```python
from build123d import *

# Parameters (mm, degrees)
EXTRUDE_1_DEPTH     = 3
SKETCH_2_W          = 4
SKETCH_2_H          = 25
EXTRUDE_2_DEPTH     = 3
SKETCH_6_R          = 1.6
CUT_EXTRUDE_4_DEPTH = 4
CUT_EXTRUDE_5_DEPTH = 10
CUT_EXTRUDE_7_DEPTH = 10
FILLET_1_R          = 5
SKETCH_11_R         = 1.5
CUT_EXTRUDE_8_DEPTH = 90.117899437


with BuildPart() as part:
    # 草图1 → 凸台-拉伸1 (new body)
    with BuildSketch(Plane(origin=(0, 0, 0), x_dir=(0, 0, -1), z_dir=(1, 0, 0))):
        Polygon((-46, -23), (-68, 40), (-74, 40), (-74, -20.726707409), (-61, -40), (-61, -43), (-31, -43), (-31, -40), (19, -40), (19, -43), (49, -43), (49, -40), (74, -2.935975787), (74, 40), (68, 40), (34, -23), align=None)
    extrude(amount=EXTRUDE_1_DEPTH)

    # 草图2 → 凸台-拉伸2 (add)
    with BuildSketch(Plane(origin=(3, 0, 0), x_dir=(0, 0, -1), z_dir=(1, 0, 0))):
        with Locations((-76, 17.5)):
            Rectangle(SKETCH_2_W, SKETCH_2_H)
        with Locations((76, 17.5)):
            Rectangle(SKETCH_2_W, SKETCH_2_H)
    extrude(amount=-EXTRUDE_2_DEPTH)

    # 草图6 → 切除-拉伸4 (cut)
    with BuildSketch(Plane.ZY):
        with Locations((-71, 5)):
            Circle(SKETCH_6_R)
        with Locations((71, 25)):
            Circle(SKETCH_6_R)
        with Locations((71, 5)):
            Circle(SKETCH_6_R)
        with Locations((-71, 25)):
            Circle(SKETCH_6_R)
    extrude(amount=-CUT_EXTRUDE_4_DEPTH, mode=Mode.SUBTRACT)

    # 草图7 → 切除-拉伸5 (cut)
    with BuildSketch(Plane(origin=(3, 0, 0), x_dir=(0, 0, -1), z_dir=(1, 0, 0))):
        with BuildLine():
            Line((-66, 13.209781141), (-66, -4.624153975))
            ThreePointArc((-66, -4.624153975), (-65.936068557, -4.975971621), (-65.752448687, -5.282804848))
            Line((-65.752448687, -5.282804848), (-55.391275304, -17.119502604))
            ThreePointArc((-55.391275304, -17.119502604), (-54.135455337, -17.324921956), (-53.694734868, -16.131168898))
            Line((-53.694734868, -16.131168898), (-64.055908251, 13.539463974))
            ThreePointArc((-64.055908251, 13.539463974), (-65.167194873, 14.195705009), (-66, 13.209781141))
        make_face()
        with BuildLine():
            Line((66, -4.449930151), (66, 21.807804944))
            ThreePointArc((66, 21.807804944), (65.244926343, 22.777346633), (64.119977827, 22.282737545))
            Line((64.119977827, 22.282737545), (42.579599238, -17.630316899))
            ThreePointArc((42.579599238, -17.630316899), (42.777733508, -18.836706189), (43.995039468, -18.94983668))
            Line((43.995039468, -18.94983668), (65.535418057, -5.29451733))
            ThreePointArc((65.535418057, -5.29451733), (65.876190064, -4.931895887), (66, -4.449930151))
        make_face()
        Polygon((-74, 0), (-61, -40), (-74, -20.726707409), align=None)
        with BuildLine():
            Line((-62.213350607, -13.880667443), (-52.307335811, -25.197387929))
            ThreePointArc((-52.307335811, -25.197387929), (-52.061835208, -25.920048281), (-52.39764858, -26.605422566))
            Line((-52.39764858, -26.605422566), (-57.236264859, -30.880697516))
            ThreePointArc((-57.236264859, -30.880697516), (-58.161708676, -31.096025601), (-58.849434846, -30.440399824))
            Line((-58.849434846, -30.440399824), (-63.916833363, -14.848404388))
            ThreePointArc((-63.916833363, -14.848404388), (-63.459750443, -13.669828659), (-62.213350607, -13.880667443))
        make_face()
        with BuildLine():
            Line((-55.387669494, -33.250616236), (-49.831358953, -28.341205383))
            ThreePointArc((-49.831358953, -28.341205383), (-49.414538234, -28.121145774), (-48.943216882, -28.116463272))
            Line((-48.943216882, -28.116463272), (-27.782801194, -33.025874126))
            ThreePointArc((-27.782801194, -33.025874126), (-27.015296935, -34.11374121), (-28.008807346, -35))
            Line((-28.008807346, -35), (-54.725533576, -35))
            ThreePointArc((-54.725533576, -35), (-55.660783212, -34.353988867), (-55.387669494, -33.250616236))
        make_face()
        with BuildLine():
            Line((-23.126212383, -29), (11.126212383, -29))
            ThreePointArc((11.126212383, -29), (12.119722794, -29.88625879), (11.352218536, -30.974125874))
            Line((11.352218536, -30.974125874), (-5.773993847, -34.947564496))
            ThreePointArc((-5.773993847, -34.947564496), (-6, -34.973438622), (-6.226006153, -34.947564496))
            Line((-6.226006153, -34.947564496), (-23.352218536, -30.974125874))
            ThreePointArc((-23.352218536, -30.974125874), (-24.119722794, -29.88625879), (-23.126212383, -29))
        make_face()
        with BuildLine():
            Line((15.782801194, -33.025874126), (36.943216882, -28.116463272))
            ThreePointArc((36.943216882, -28.116463272), (37.414538234, -28.121145774), (37.831358953, -28.341205383))
            Line((37.831358953, -28.341205383), (43.387669494, -33.250616236))
            ThreePointArc((43.387669494, -33.250616236), (43.660783212, -34.353988867), (42.725533576, -35))
            Line((42.725533576, -35), (16.008807346, -35))
            ThreePointArc((16.008807346, -35), (15.015296935, -34.11374121), (15.782801194, -33.025874126))
        make_face()
        with BuildLine():
            Line((40.32049134, -24.831312908), (58.783941471, -13.126583263))
            ThreePointArc((58.783941471, -13.126583263), (60.036438838, -13.274178861), (60.148397101, -14.530363346))
            Line((60.148397101, -14.530363346), (48.30691143, -32.086087811))
            ThreePointArc((48.30691143, -32.086087811), (47.604393348, -32.518859029), (46.815737939, -32.276278671))
            Line((46.815737939, -32.276278671), (40.193773479, -26.425283852))
            ThreePointArc((40.193773479, -26.425283852), (39.859054482, -25.596651891), (40.32049134, -24.831312908))
        make_face()
    extrude(amount=-CUT_EXTRUDE_5_DEPTH, mode=Mode.SUBTRACT)

    # 草图10 → 切除-拉伸7 (cut)
    with BuildSketch(Plane.ZY):
        with BuildLine():
            Line((61.096725602, -39.702382762), (61, -40.312940669))
            ThreePointArc((61, -40.312940669), (61, -40), (61.096725602, -39.702382762))
        make_face()
        with BuildLine():
            Line((-74, 30), (-74, 32))
            ThreePointArc((-74, 32), (-73, 31), (-74, 30))
        make_face()
        with BuildLine():
            Line((74, 30), (74, 32))
            ThreePointArc((74, 32), (73, 31), (74, 30))
        make_face()
        with BuildLine():
            Line((-74, 3.585786438), (-75.414213562, 5))
            ThreePointArc((-75.414213562, 5), (-74, 5), (-74, 3.585786438))
        make_face()
        with BuildLine():
            Line((74, 3.585786438), (75.414213562, 5))
            ThreePointArc((75.414213562, 5), (74, 5), (74, 3.585786438))
        make_face()
        with BuildLine():
            Line((-17, -40), (-19, -40))
            ThreePointArc((-19, -40), (-18, -39), (-17, -40))
        make_face()
        with BuildLine():
            Line((29, -40), (31, -40))
            ThreePointArc((31, -40), (30, -39), (29, -40))
        make_face()
        with BuildLine():
            Line((-49.326984365, -39.515225743), (-49, -40.584743409))
            ThreePointArc((-49, -40.584743409), (-49, -40), (-49.326984365, -39.515225743))
        make_face()
    extrude(amount=-CUT_EXTRUDE_7_DEPTH, mode=Mode.SUBTRACT)

    # 圆角1
    fillet_1_edges = [part.edges().sort_by_distance(p)[0] for p in [
        (1.5, -23, 46),
        (1.5, -23, -34),
    ]]
    fillet(fillet_1_edges, radius=FILLET_1_R)

    # 草图11 → 切除-拉伸8 (cut, through all)
    with BuildSketch(Plane(origin=(3, 0, 0), x_dir=(0, 0, -1), z_dir=(1, 0, 0))):
        with Locations((-1, -26)):
            Circle(SKETCH_11_R)
        with Locations((-21, -26)):
            Circle(SKETCH_11_R)
    extrude(amount=-CUT_EXTRUDE_8_DEPTH, mode=Mode.SUBTRACT)


solid = part.part
```
Work out the finished part from the listing and answer in its coordinate system (mm). A direction names the side the tool comes from. Coordinates: 2 decimals unless noted, no trailing zeros. Loops run counter-clockwise (first coordinate to the right, second up) from the corner with the lowest first, then second, coordinate; pieces in that order, holes last. Notation, with made-up numbers: (29.5, -22.5) - (37.5, -22.5) arc R14 ccw to (37.5, 1.5) - close; hole circle Ø5 at (84, 74). An arc over 180 degrees is marked (long way). Use a Markdown table: item, result.
Item 1: For faces 1 (the cylindrical face through (1.52, -22.05, 45.38)), 2 (the flat face through (2, 30, -76)), 3 (the flat face through (1, 0, -74)), 4 (the flat face through (1.521, -30.606, -26.215)), 5 (the flat face through (2, 30, 76)), determine the directions among +Z, -Z, +X, -X, +Y, -Y from which every point of the face is accessible in a straight line to the end or side of a thin tool.
Evaluation:
| item | result |
|---|---|
| face 1 | +X, -X, +Y |
| face 2 | -Z, +X, -X, +Y |
| face 3 | -Z, +X, -X, -Y |
| face 4 | +X, -X |
| face 5 | +Z, +X, -X, +Y |
Item 2: Consider probe 1 along Z at (x, y) = (1.75, 16); probe 2 along Y at (x, z) = (1.85, -71); probe 3 along Y at (x, z) = (1.15, -37). Determine where each line is inside the solid, lowest interval first. Write a range as from..to.
Evaluation:
| item | result |
|---|---|
| probe 1 | z = -78..-66, -60.73..-55.05, 59.62..78 |
| probe 2 | y = -7.38..3.4, 6.6..23.4, 26.6..40 |
| probe 3 | y = -43..-35, -28.11..-17.44 |
Item 3: Find section C-C, the plane x = 0.7. State how many separate pieces and enclosed holes the cut face has, and give its area (3 significant figures).
Evaluation:
| item | result |
|---|---|
| separate pieces | 1 |
| enclosed holes | 13 |
| area | 3,470 mm2 |
Item 4: Find section A-A, the plane z = -56.5. Determine the outline of the cut face in (x, y), and give its area (3 significant figures).
Evaluation:
| item | result |
|---|---|
| outline | (0, -28.88) - (3, -28.88) - (3, -19.94) - (0, -19.94) - close; (0, -14.57) - (3, -14.57) - (3, -11.02) - (0, -11.02) - close; (0, 8.16) - (3, 8.16) - (3, 18.69) - (0, 18.69) - close |
| area | 69.1 mm2 |
Item 5: Given pin 1 Ø0.9 at (x, z) = (1.5, 10.5) entering from -Y; pin 2 Ø0.8 at (x, y) = (1, -41.5) entering from +Z; pin 3 Ø0.9 at (x, y) = (1, 1.5) entering from -Z; pin 4 Ø1.9 at (y, z) = (5, 71) entering from -X, each flat-ended and moving along its own axis, determine where each tip first touches the part or whether it passes through.
Evaluation:
| item | result |
|---|---|
| pin 1 | stops at y = -40 |
| pin 2 | stops at z = 61 |
| pin 3 | stops at z = -74 |
| pin 4 | passes through |
Item 6: Find section B-B, the plane z = 10.5. Determine the outline of the cut face in (x, y).
Evaluation:
| item | result |
|---|---|
| outline | (0, -40) - (3, -40) - (3, -33.96) - (0, -33.96) - close; (0, -29) - (3, -29) - (3, -23) - (0, -23) - close |
Item 7: Find section D-D, the plane z = 71. Determine the outline of the cut face in (x, y).
Evaluation:
| item | result |
|---|---|
| outline | (0, -9.23) - (3, -9.23) - (3, 3.4) - (0, 3.4) - close; (0, 6.6) - (3, 6.6) - (3, 23.4) - (0, 23.4) - close; (0, 26.6) - (3, 26.6) - (3, 40) - (0, 40) - close |
